The drawing under review shows one solid part. Ordinate dimensions are in mm from its lowest x, y, z. A direction names the side the tool comes from. Coordinates: 2 decimals unless noted, no trailing zeros. Loops run counter-clockwise (first coordinate to the right, second up) from the corner with the lowest first, then second, coordinate; pieces in that order, holes last. Notation, with made-up numbers: (40, -38) - (57, -38) arc R25 ccw to (57, -2) - close; hole circle Ø2 at (84, -10.5). An arc over 180 degrees is marked (long way). Use one line per item in the form item = value. Start each with the question number.
1. Add section D-D on x = 7.5. Give the boundary of the cut face in (y, z).
2. For pin 1 Ø1 at (x, z) = (8, 3.5) entering from -Y; pin 2 Ø2 at (x, y) = (8, 13.5) entering from +Z; pin 3 Ø3 at (x, z) = (4, 7) entering from -Y, all flat-tipped, find the tip position at first contact; note any pin that passes through.
3. Machinability: for the marked faces 1 and 2, which of the approach directions +Z, -Z, +X, -X, +Y, -Y give a long, thin tool a straight path to every point of the face, cutting with its end or side? Answer none if there is none.
4. Draft analysis for pull direction X (two halves, no side actions). For the marked faces 3, 4 and 5, state which applies: +X half, -X half, draft (parallel to the pull), parting line (faces both ways), or undercut.
5. Add section C-C on x = 6.25. Give the boundary of the cut face in (y, z).
6. Add section B-B on z = 2.5. Give the boundary of the cut face in (x, y).
7. Add section A-A on y = 14.75. Give the boundary of the cut face in (x, z), and give its area (3 significant figures).
8. To check wall thickness, follow probe 1 along Z at (x, y) = (9, 8); probe 2 along X at (y, z) = (8.5, 3.25). State the ranges of each line that lie inside material, in increasing order.
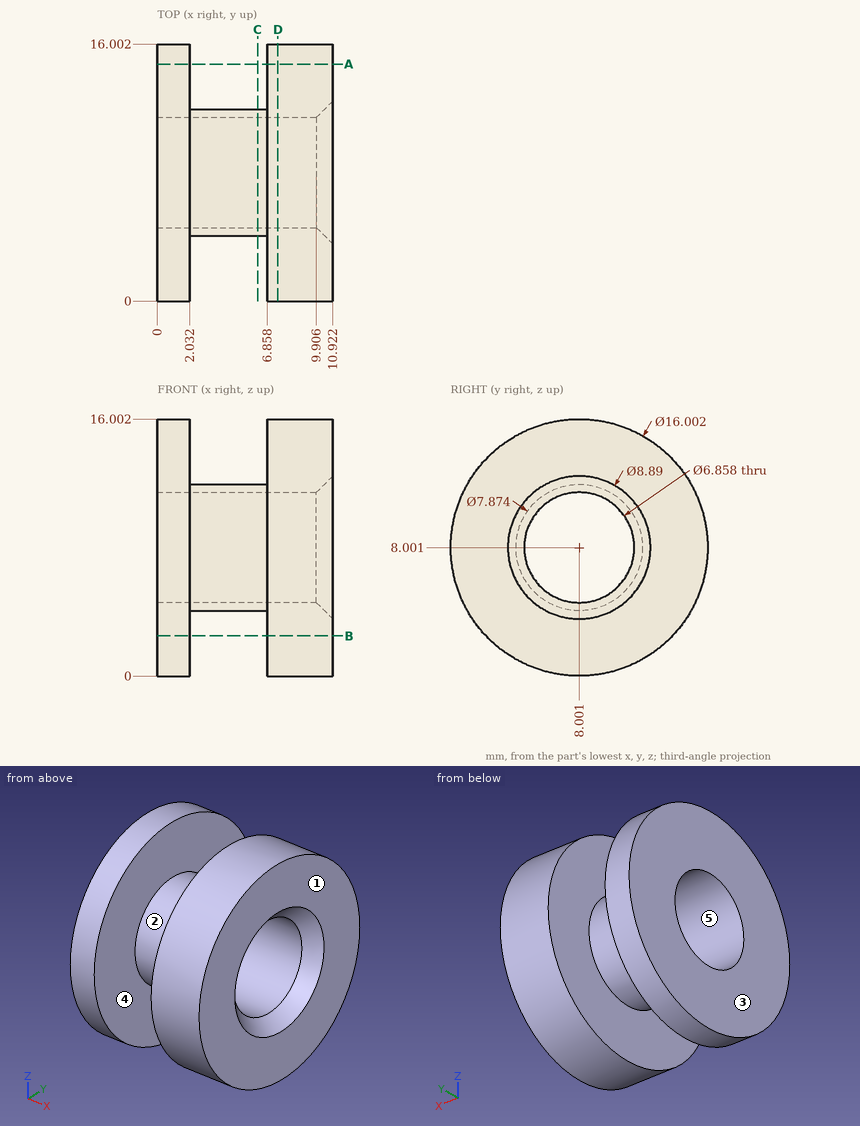
Conclusion:
q1.outline = circle Ø16 at (8, 8); hole circle Ø6.86 at (8, 8)
q2.pin_1 = 1.07
q2.pin_2 = 14.62
q2.pin_3 = 4.06
q3.face_1 = +Z, -Z, +X, +Y, -Y
q3.face_2 = none
q4.face_3 = -X half
q4.face_4 = undercut
q4.face_5 = draft
q5.outline = circle Ø7.87 at (8, 8); hole circle Ø6.86 at (8, 8)
q6.outline = (0, 2.19) - (2.03, 2.19) - (2.03, 13.81) - (0, 13.81) - close; (6.86, 2.19) - (10.92, 2.19) - (10.92, 13.81) - (6.86, 13.81) - close
q7.outline = (0, 3.7) - (2.03, 3.7) - (2.03, 12.3) - (0, 12.3) - close; (6.86, 3.7) - (10.92, 3.7) - (10.92, 12.3) - (6.86, 12.3) - close
q7.area = 52.4 mm^2
q8.probe_1 = 0 to 4.57, 11.43 to 16
q8.probe_2 = 0 to 2.03, 6.86 to 10.92
